The listing builds one solid part. Answer for the finished solid, in the listing's coordinates (mm). Coordinates: 2 decimals unless noted, no trailing zeros. Order: outer loops, then holes, each group sorted by start corner. A loop starts at its lowest first (then second) coordinate and runs counter-clockwise, first axis right, second up.
```python
from build123d import *

# Parameters (mm, degrees)
SKETCH1_W                       = 58
SKETCH1_H                       = 35
BOSS_EXTRUDE1_DEPTH             = 2
M3X0_5_TAPPED_HOLE1_D           = 2.5
M3X0_5_TAPPED_HOLE1_CSINK_D     = 3.05
M3X0_5_TAPPED_HOLE1_CSINK_ANGLE = 90
CUT_EXTRUDE1_DEPTH              = 34.930075155
CHAMFER1_SIZE                   = 2


with BuildPart() as part:
    # Sketch1 → Boss-Extrude1 (new body)
    with BuildSketch(Plane(origin=(0, 0, 0), x_dir=(1, 0, 0), z_dir=(0, 1, 0))):
        Rectangle(SKETCH1_W, SKETCH1_H)
    extrude(amount=BOSS_EXTRUDE1_DEPTH)

    # M3x0.5 Tapped Hole1 (through all)
    with Locations(Plane(origin=(0, 2, 0), x_dir=(1, 0, 0), z_dir=(0, 1, 0))):
        with Locations((-23, 12.5), (-3, 12.5), (16.8, 12.5), (16.8, -6.5), (-23, -1.5)):
            CounterSinkHole(M3X0_5_TAPPED_HOLE1_D / 2, M3X0_5_TAPPED_HOLE1_CSINK_D / 2, counter_sink_angle=M3X0_5_TAPPED_HOLE1_CSINK_ANGLE)

    # Sketch4 → Cut-Extrude1 (cut, through all)
    with BuildSketch(Plane(origin=(0, 2, 0), x_dir=(1, 0, 0), z_dir=(0, 1, 0))):
        with BuildLine():
            ThreePointArc((-8.204545455, -3.514584349), (-11.5, -6.5), (-8.204545455, -9.485415651))
            ThreePointArc((-8.204545455, -9.485415651), (3, -6.5), (-8.204545455, -3.514584349))
        make_face()
    extrude(amount=-CUT_EXTRUDE1_DEPTH, mode=Mode.SUBTRACT)

    # Chamfer1
    chamfer1_edges = [part.edges().sort_by_distance(p)[0] for p in [
        (29, 1, 17.5),
        (-29, 1, 17.5),
        (-29, 1, -17.5),
        (29, 1, -17.5),
    ]]
    chamfer(chamfer1_edges, length=CHAMFER1_SIZE)


solid = part.part
```
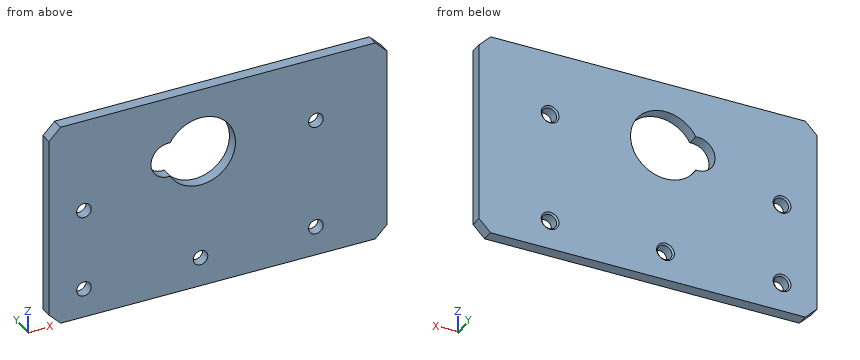
1) A cutting plane is placed at A-A, the plane x = -3. Write down the section's boundary in (y, z) (3 decimals), plus the area to 3 significant figures.
2) A cutting plane is placed at C-C, the plane z = 1.5. Write down the section's boundary in (x, y) (3 decimals), plus the area to 3 significant figures.
3) Each of these flat-tipped pins is pushed along its axis until it touches: P1, Ø15.5, axis at x = -3, z = 6.5, coming from the -Y side; P2, Ø2, axis at x = 16.8, z = 6.5, coming from the +Y side. Where does it stop, or does it pass through?
4) A cutting plane is placed at D-D, the plane x = -23. Write down the section's boundary in (y, z) (3 decimals).
5) Straight lines are drawn through the part: probe 1 along Z at (x, y) = (-3, 0.75); probe 2 along Z at (x, y) = (16.8, 0.7); probe 3 along X at (y, z) = (0.6, -12.5). For each, find the intervals that lie inside material, in ascending order.
6) A cutting plane is placed at B-B, the plane y = 1.4. Write down the section's boundary in (x, z), plus the area to 3 significant figures.
Working result:
1. outline: (0, -17.5) - (2, -17.5) - (2, -14.025) - (1.725, -13.75) - (0, -13.75) - close; (0, -11.25) - (1.725, -11.25) - (2, -10.975) - (2, 0.5) - (0, 0.5) - close; (0, 12.5) - (2, 12.5) - (2, 17.5) - (0, 17.5) - close
1. area: 40.9 mm2
2. outline: (-29, 0) - (-24.25, 0) - (-24.25, 1.725) - (-24.525, 2) - (-29, 2) - close; (-21.75, 0) - (-6.317, 0) - (-6.317, 2) - (-21.475, 2) - (-21.75, 1.725) - close; (0.317, 0) - (29, 0) - (29, 2) - (0.317, 2) - close
2. area: 97.7 mm2
3. P1: stops at y = 0
3. P2: passes through
4. outline: (0, -17.5) - (2, -17.5) - (2, -14.025) - (1.725, -13.75) - (0, -13.75) - close; (0, -11.25) - (1.725, -11.25) - (2, -10.975) - (2, -0.025) - (1.725, 0.25) - (0, 0.25) - close; (0, 2.75) - (1.725, 2.75) - (2, 3.025) - (2, 17.5) - (0, 17.5) - close
5. probe 1: z = -17.5 to -13.75, -11.25 to 0.5, 12.5 to 17.5
5. probe 2: z = -17.5 to -13.75, -11.25 to 5.25, 7.75 to 17.5
5. probe 3: x = -29 to -24.25, -21.75 to -4.25, -1.75 to 15.55, 18.05 to 29
6. outline: (-29, -15.5) - (-27, -17.5) - (27, -17.5) - (29, -15.5) - (29, 15.5) - (27, 17.5) - (-27, 17.5) - (-29, 15.5) - close; hole circle Ø2.5 at (-23, -12.5); hole circle Ø2.5 at (-23, 1.5); hole (-8.2, 3.51) arc R6 ccw (long way) to (-8.2, 9.49) arc R3 ccw (long way) to start; hole circle Ø2.5 at (-3, -12.5); hole circle Ø2.5 at (16.8, -12.5); hole circle Ø2.5 at (16.8, 6.5)
6. area: 1,870 mm2
